from build123d import *

# Parameters (mm, degrees)
EXTRUDE_1_DEPTH = 2
EXTRUDE_START   = -3
EXTRUDE_2_DEPTH = 3
SKETCH_4_W      = 3
SKETCH_4_H      = 3
EXTRUDE_3_DEPTH = 40
SKETCH_6_W      = 3
SKETCH_6_H      = 3
EXTRUDE_4_DEPTH = 3
FILLET_1_R      = 1


with BuildPart() as part:
    # 草图1 → 旋转1 (revolve)
    with BuildSketch(Plane.XY, mode=Mode.PRIVATE) as revolve_1_sk:
        Polygon((-2.4, 0), (-3.5, 0), (-3.5, 5), (-2.25, 5), (-2.25, 3.8), (-1.25, 3.8), (-1.25, 2.66), (-2.4, 2.66), align=None)
    revolve(revolve_1_sk.sketch.rotate(Axis((0, 0, 0), (0, 1, 0)), 270), axis=Axis((0, 0, 0), (0, 1, 0)))

    # 草图2 → 凸台-拉伸1 (add)
    with BuildSketch(Plane(origin=(0, 2, 0), x_dir=(-1, 0, 0), z_dir=(0, -1, 0))):
        with BuildLine():
            Line((-3.493157374, 0.21875), (-3.493157374, 5.21875))
            Line((-3.493157374, 5.21875), (3.493157374, 5.21875))
            Line((3.493157374, 5.21875), (3.493157374, 0.21875))
            ThreePointArc((3.493157374, 0.21875), (0, 3.5), (-3.493157374, 0.21875))
        make_face()
    extrude(amount=EXTRUDE_1_DEPTH)

    # 草图2<2> → 凸台-拉伸2 (add)
    with BuildSketch(Plane(origin=(0, 2, 0), x_dir=(-1, 0, 0), z_dir=(0, -1, 0)).offset(EXTRUDE_START)):
        with BuildLine():
            Line((-3.493157374, 0.21875), (-3.493157374, 5.21875))
            Line((-3.493157374, 5.21875), (3.493157374, 5.21875))
            Line((3.493157374, 5.21875), (3.493157374, 0.21875))
            ThreePointArc((3.493157374, 0.21875), (0, 3.5), (-3.493157374, 0.21875))
        make_face()
    extrude(amount=EXTRUDE_2_DEPTH)

    # 草图4 → 凸台-拉伸3 (add)
    with BuildSketch(Plane(origin=(0, 0, -5.21875), x_dir=(-1, 0, 0), z_dir=(0, 0, -1))):
        with Locations((0, 2)):
            Rectangle(SKETCH_4_W, SKETCH_4_H)
    extrude(amount=EXTRUDE_3_DEPTH)

    # 草图6 → 凸台-拉伸4 (add)
    with BuildSketch(Plane(origin=(0, 0, -45.21875), x_dir=(-1, 0, 0), z_dir=(0, 0, -1))):
        with Locations((0, 2)):
            Rectangle(SKETCH_6_W, SKETCH_6_H)
    extrude(amount=EXTRUDE_4_DEPTH)

    # 圆角1
    fillet_1_edges = [part.edges().sort_by_distance(p)[0] for p in [
        (-1.5, 0.5, -26.71875),
        (-1.5, 3.5, -26.71875),
        (1.5, 3.5, -26.71875),
        (1.5, 0.5, -26.71875),
    ]]
    fillet(fillet_1_edges, radius=FILLET_1_R)


solid = part.part
Here's how the part is built. I have some questions about the finished solid (model axes, mm). A direction names the side the tool comes from. Round coordinates to 2 decimals unless told otherwise and drop trailing zeros. Loops run counter-clockwise (first coordinate to the right, second up) from the corner with the lowest first, then second, coordinate; pieces in that order, holes last. Notation, with made-up numbers: (57, 4.25) - (82, 4.25) arc R20 cw to (82, 11.25) - close; hole circle Ø4 at (45, 78). An arc over 180 degrees is marked (long way). One line per question, with ' | ' between items. Start each with the question number.
Q1. For faces 1 (the cylindrical face through (1.215, 0.801, -27.02)), 2 (the cylindrical face through (-0.676, 4.392, -2.146)), 3 (the flat face through (0, 3.5, -26)), 4 (the cylindrical face through (1.215, 3.199, -26.418)), which set-ups out of +Z, -Z, +X, -X, +Y, -Y let a thin tool reach every point of the face, with its end or its side?
Q2. I want a section at B-B (z = -13). Write out the boundary of the cut face in (x, y), then the cut area to 3 significant figures.
Q3. I want a section at A-A (x = 0). Write out the boundary of the cut face in (y, z).
Q4. Please list where these lines run through material, in increasing order: line 1 (X direction, y = 1.5, z = 0); line 2 (X direction, y = 4.5, z = 0); line 3 (X direction, y = 1.35, z = -20). Write a range as [from, to].
Q5. We'd pull the mould along X, two halves only. Please class faces 5 (the cylindrical face through (-1.215, 3.199, -26.418)), 6 (the flat face through (0, 0, -3)), 7 (the cylindrical face through (-2.024, 1.311, -1.29)): +X half, -X half, draft (parallel to the pull), parting line (faces both ways), or undercut.
Q6. Will these pins go through, and if not, where does the flat tip stop? pin 1 (1.5 mm diameter, centred on y = 3.5, z = -1.5, fed in from +X); pin 2 (1 mm diameter, centred on x = -2.5, y = 2.5, fed in from +Z); pin 3 (2.5 mm diameter, centred on x = 0, z = 0.5, fed in from -Y); pin 4 (1.5 mm diameter, centred on x = 0, z = 0, fed in from -Y).
Response values:
1) face 1: -Z, +X, -Y | face 2: +Y | face 3: -Z, +X, -X, +Y | face 4: -Z, +X, +Y
2) outline: (-1.5, 1.5) arc R1 ccw to (-0.5, 0.5) - (0.5, 0.5) arc R1 ccw to (1.5, 1.5) - (1.5, 2.5) arc R1 ccw to (0.5, 3.5) - (-0.5, 3.5) arc R1 ccw to (-1.5, 2.5) - close | area: 8.14 mm²
3) outline: (0, -5.22) - (0.5, -5.22) - (0.5, -48.22) - (3.5, -48.22) - (3.5, -5.22) - (5, -5.22) - (5, -2.25) - (3.8, -2.25) - (3.8, -1.25) - (2.66, -1.25) - (2.66, -2.4) - (0, -2.4) - close; (0, 2.4) - (2.66, 2.4) - (2.66, 1.25) - (3.8, 1.25) - (3.8, 2.25) - (5, 2.25) - (5, 3.5) - (0, 3.5) - close
4) line 1: x = [-3.5, -2.4], [2.4, 3.5] | line 2: x = [-3.5, -2.25], [2.25, 3.5] | line 3: x = [-1.49, 1.49]
5) face 5: -X half | face 6: draft | face 7: undercut
6) pin 1: stops at x = 3.49 | pin 2: stops at z = 2.87 | pin 3: stops at y = 2.66 | pin 4: passes through
